Geometry check sheet. Reference: the model listing, model coordinates, mm. Round coordinates to 2 decimals unless told otherwise and drop trailing zeros. Order: outer loops, then holes, each group sorted by start corner. A loop starts at its lowest first (then second) coordinate and runs counter-clockwise, first axis right, second up.
(1) Cross-section at C-C on z = -12. Enter the section's corners in (x, y).
(2) Thickness scan on L1, parallel to Y at x = 0, z = -24; L2, parallel to Y at x = 2, z = 9; L3, parallel to X at y = -0.95, z = 26. Record the ranges inside material, lowest first.
(3) Gauge pin test, flat ends, axial feed: P1, Ø1.5, axis at x = 0.5, z = 13.5, coming from the +Y side; P2, Ø2.5, axis at x = 0, y = 0, coming from the +Z side; P3, Ø1, axis at x = 1, z = 5, coming from the -Y side; P4, Ø0.8, axis at x = 0, y = 0, coming from the -Z side. Record the tip position at first contact, or that the pin passes through.
(4) Cross-section at A-A on x = 0. Enter the section's corners in (y, z), and give its area (3 significant figures).
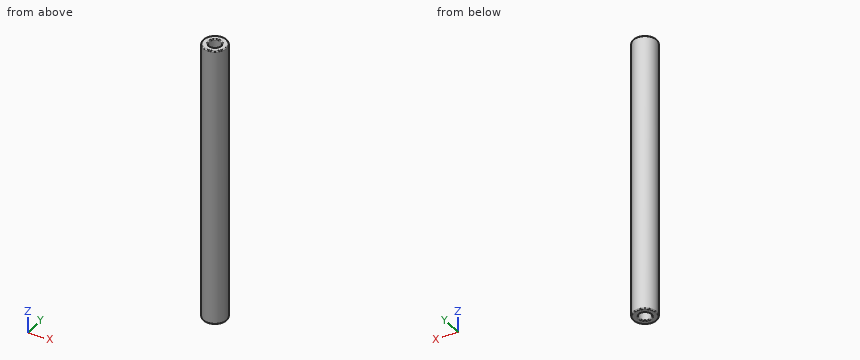
from build123d import *

# Parameters (mm, degrees)
F0_R     = 2.5
F1_DEPTH = 30
F2_R     = 1.3
F3_DEPTH = 10
F4_R     = 1.3
F5_DEPTH = 10
F6_R     = 0.2


with BuildPart() as f1:
    # F0 (on Top) → F1 (new body, symmetric)
    with BuildSketch(Plane.XY):
        Circle(F0_R)
    extrude(amount=F1_DEPTH, both=True)

    # F2 (on face) → F3 (cut)
    with BuildSketch(Plane.XY.offset(30)):
        Circle(F2_R)
    extrude(amount=-F3_DEPTH, mode=Mode.SUBTRACT)

    # F4 (on face) → F5 (cut)
    with BuildSketch(Plane(origin=(0, 0, -30), x_dir=(1, 0, 0), z_dir=(0, 0, -1))):
        Circle(F4_R)
    extrude(amount=-F5_DEPTH, mode=Mode.SUBTRACT)

    # F6
    f6_edges = [f1.edges().sort_by_distance(p)[0] for p in [
        (-2.5, 0, -30),
        (-1.3, 0, -30),
        (-2.5, 0, 30),
        (-1.3, 0, 30),
    ]]
    fillet(f6_edges, radius=F6_R)


solid = f1.part
Found:
1. outline: circle Ø5 at (0, 0)
2. L1: y = -2.5 to -1.3, 1.3 to 2.5
2. L2: y = -1.5 to 1.5
2. L3: x = -2.31 to -0.89, 0.89 to 2.31
3. P1: stops at y = 2.5
3. P2: stops at z = 20
3. P3: stops at y = -2.45
3. P4: stops at z = -20
4. outline: (-2.5, -29.8) arc R0.2 ccw to (-2.3, -30) - (-1.5, -30) arc R0.2 ccw to (-1.3, -29.8) - (-1.3, -20) - (1.3, -20) - (1.3, -29.8) arc R0.2 ccw to (1.5, -30) - (2.3, -30) arc R0.2 ccw to (2.5, -29.8) - (2.5, 29.8) arc R0.2 ccw to (2.3, 30) - (1.5, 30) arc R0.2 ccw to (1.3, 29.8) - (1.3, 20) - (-1.3, 20) - (-1.3, 29.8) arc R0.2 ccw to (-1.5, 30) - (-2.3, 30) arc R0.2 ccw to (-2.5, 29.8) - close
4. area: 248 mm2
